The listing builds one solid part. Answer for the finished solid, in the listing's coordinates (mm). A direction names the side the tool comes from. Give positions to 0.01 mm unless a question says otherwise; leave off trailing zeros. Write each loop counter-clockwise with the first axis right and the second up, starting at its lowest first coordinate (ties: lowest second). Pieces come first, ordered by that corner, then holes. Notation, with made-up numbers: (-32.5, 61) - (-8.5, 61) arc R29 cw to (-8.5, 99) - close; hole circle Ø7 at (59.25, -10). An arc over 180 degrees is marked (long way). Write each question's results on one line, items separated by ' | '. Start each with the question number.
Q1. Flat-ended cylindrical pins translate along their axes: pin 1 Ø3 at (y, z) = (16, -15.5) entering from -X (3 decimals); pin 2 Ø2 at (y, z) = (-15.5, 15.5) entering from +X (3 decimals); pin 3 Ø3 at (y, z) = (21.68, -37.54) entering from -X; pin 4 Ø14.5 at (y, z) = (0, 0) entering from -X. Find the tip coordinate at first contact, or state that the pin passes through.
Q2. For faces 1 (the face through (2.18, 0.53, -11.99)), 2 (the face through (-7.225, -6, 12)), 3 (the face through (11.336, -28.203, 36.782)), determine the directions among +Z, -Z, +X, -X, +Y, -Y from which every point of the face is accessible in a straight line to the end or side of a thin tool.
Q3. Section A-A (y = 0) is taken. Determine the outline of the cut face in (x, z) (3 decimals).
Q4. Section B-B (x = 5.5) is taken. Determine the outline of the cut face in (y, z), plus the area to 3 significant figures.
Q5. Find the intervals of material crossed by probe 1 along Y at (x, z) = (4, 0); probe 2 along Y at (x, z) = (11.5, 0); probe 3 along X at (y, z) = (-7, -15) (3 decimals), in increasing order.
```python
from build123d import *

# Parameters (mm, degrees)
SKETCH1_R                    = 48.35
BOSS_EXTRUDE1_DEPTH          = 12.575
SKETCH2_R                    = 1.25
CUT_EXTRUDE1_DEPTH           = 3
CHAMFER1_SIZE                = 0.5
CIRPATTERN1_COUNT            = 6
CHAMFER1_OF_CIRPATTERN1_SIZE = 0.5
SKETCH3_R                    = 12
CUT_EXTRUDE2_DEPTH           = 25.15
CHAMFER2_SIZE                = 1.25
CHAMFER3_SIZE                = 0.5
SKETCH4_R                    = 28.25
CUT_EXTRUDE3_DEPTH           = 5.35
SKETCH5_R                    = 3.5
BOSS_EXTRUDE2_DEPTH          = 3.85
SKETCH6_R                    = 1.25
CUT_EXTRUDE4_DEPTH           = 5.85
SKETCH7_R                    = 46.35
CUT_EXTRUDE5_DEPTH           = 2
SKETCH8_R                    = 48.35
SKETCH8_R_2                  = 46.35
CUT_EXTRUDE6_DEPTH           = 0.5
CHAMFER4_SIZE                = 1.25


with BuildPart() as part:
    # Sketch1 → Boss-Extrude1 (new, symmetric)
    with BuildSketch(Plane(origin=(0, 0, 0), x_dir=(0, 0, -1), z_dir=(1, 0, 0))):
        with Locations(Location((0, 0, 0), (0, 0, 180))):
            Circle(SKETCH1_R)
    extrude(amount=BOSS_EXTRUDE1_DEPTH, both=True)

    # Sketch2 → Cut-Extrude1 (cut)
    with BuildSketch(Plane.ZY.offset(12.575)):
        with Locations((0, 43.35)):
            Circle(SKETCH2_R)
    cut_extrude1 = extrude(amount=-CUT_EXTRUDE1_DEPTH, mode=Mode.SUBTRACT)

    # Chamfer1
    chamfer1_edges = [part.edges().sort_by_distance(p)[0] for p in [
        (-12.575, 43.35, -1.25),
    ]]
    chamfer(chamfer1_edges, length=CHAMFER1_SIZE)

    # CirPattern1: Cut-Extrude1 ×6 about axis
    cirpattern1_axis = Axis((0, 0, 0), (1, 0, 0))
    for i in range(1, CIRPATTERN1_COUNT):
        add(cut_extrude1.rotate(cirpattern1_axis, i * 360 / CIRPATTERN1_COUNT), mode=Mode.SUBTRACT)

    # Chamfer1 of CirPattern1
    chamfer1_of_cirpattern1_edges = [part.edges().sort_by_distance(p)[0] for p in [
        (-12.575, 22.757531755, 36.917201254),
        (-12.575, -20.592468245, 38.167201254),
        (-12.575, -43.35, 1.25),
        (-12.575, -22.757531755, -36.917201254),
        (-12.575, 20.592468245, -38.167201254),
    ]]
    chamfer(chamfer1_of_cirpattern1_edges, length=CHAMFER1_OF_CIRPATTERN1_SIZE)

    # Sketch3 → Cut-Extrude2 (cut)
    with BuildSketch(Plane.ZY.offset(12.575)):
        Circle(SKETCH3_R)
    extrude(amount=-CUT_EXTRUDE2_DEPTH, mode=Mode.SUBTRACT)

    # Chamfer2
    chamfer2_edges = [part.edges().sort_by_distance(p)[0] for p in [
        (-12.575, 0, -12),
    ]]
    chamfer(chamfer2_edges, length=CHAMFER2_SIZE)

    # Chamfer3
    chamfer3_edges = [part.edges().sort_by_distance(p)[0] for p in [
        (-12.575, 0, -48.35),
    ]]
    chamfer(chamfer3_edges, length=CHAMFER3_SIZE)

    # Sketch4 → Cut-Extrude3 (cut)
    with BuildSketch(Plane.ZY.offset(12.575)):
        Circle(SKETCH4_R)
    extrude(amount=-CUT_EXTRUDE3_DEPTH, mode=Mode.SUBTRACT)

    # Sketch5 → Boss-Extrude2 (add)
    with BuildSketch(Plane.ZY.offset(7.225)):
        with Locations(Location((-15.5, 15.5, 0), (0, 0, 180))):
            Circle(SKETCH5_R)
        with Locations(Location((15.5, 15.5, 0), (0, 0, 180))):
            Circle(SKETCH5_R)
        with Locations(Location((15.5, -15.5, 0), (0, 0, 180))):
            Circle(SKETCH5_R)
        with Locations(Location((-15.5, -15.5, 0), (0, 0, 180))):
            Circle(SKETCH5_R)
    extrude(amount=BOSS_EXTRUDE2_DEPTH)

    # Sketch6 → Cut-Extrude4 (cut)
    with BuildSketch(Plane.ZY.offset(11.075)):
        with Locations((-15.5, 15.5)):
            Circle(SKETCH6_R)
        with Locations((15.5, 15.5)):
            Circle(SKETCH6_R)
        with Locations((15.5, -15.5)):
            Circle(SKETCH6_R)
        with Locations((-15.5, -15.5)):
            Circle(SKETCH6_R)
    extrude(amount=-CUT_EXTRUDE4_DEPTH, mode=Mode.SUBTRACT)

    # Sketch7 → Cut-Extrude5 (cut)
    with BuildSketch(Plane(origin=(12.575, 0, 0), x_dir=(0, 0, -1), z_dir=(1, 0, 0))):
        Circle(SKETCH7_R)
    extrude(amount=-CUT_EXTRUDE5_DEPTH, mode=Mode.SUBTRACT)

    # Sketch8 → Cut-Extrude6 (cut)
    with BuildSketch(Plane(origin=(12.575, 0, 0), x_dir=(0, 0, -1), z_dir=(1, 0, 0))):
        with Locations(Location((0, 0, 0), (0, 0, 180))):
            Circle(SKETCH8_R)
        Circle(SKETCH8_R_2, mode=Mode.SUBTRACT)
    extrude(amount=-CUT_EXTRUDE6_DEPTH, mode=Mode.SUBTRACT)

    # Chamfer4
    chamfer4_edges = [part.edges().sort_by_distance(p)[0] for p in [
        (-7.225, 0, -12),
    ]]
    chamfer(chamfer4_edges, length=CHAMFER4_SIZE)


solid = part.part
```
Answers below:
1) pin 1: stops at x = -11.075 | pin 2: stops at x = 10.575 | pin 3: stops at x = -12.33 | pin 4: passes through
2) face 1: +X, -X | face 2: -X | face 3: +X
3) outline: (-12.575, -47.85) - (-12.075, -48.35) - (12.075, -48.35) - (12.075, -46.35) - (10.575, -46.35) - (10.575, -12) - (-5.975, -12) - (-7.225, -13.25) - (-7.225, -28.25) - (-12.575, -28.25) - close; (-12.575, 28.25) - (-7.225, 28.25) - (-7.225, 13.25) - (-5.975, 12) - (10.575, 12) - (10.575, 46.35) - (12.075, 46.35) - (12.075, 48.35) - (-12.075, 48.35) - (-12.575, 47.85) - close
4) outline: circle Ø96.7 at (0, 0); hole circle Ø24 at (0, 0) | area: 6,890 mm2
5) probe 1: y = -48.35 to -12, 12 to 48.35 | probe 2: y = -48.35 to -46.35, 46.35 to 48.35 | probe 3: x = -7.225 to 10.575
